from build123d import *

# Parameters (mm, degrees)
SKETCH1_W           = 87.952115464
SKETCH1_H           = 84
BOSS_EXTRUDE1_DEPTH = 44
CUT_EXTRUDE1_DEPTH  = 105.526999639
CUT_EXTRUDE2_DEPTH  = 94
BOSS_EXTRUDE2_DEPTH = 5
CUT_EXTRUDE4_DEPTH  = 108.023520294
BOSS_EXTRUDE3_DEPTH = 89
SKETCH12_W          = 66.643398472
SKETCH12_H          = 89
CUT_EXTRUDE5_DEPTH  = 21
SKETCH13_W          = 89
SKETCH13_H          = 4.850314153
CUT_EXTRUDE6_DEPTH  = 15
SKETCH14_R          = 9.5
CUT_EXTRUDE7_DEPTH  = 67.996371003
SKETCH15_R          = 4
SKETCH15_R_2        = 1.5
BOSS_EXTRUDE4_DEPTH = 5.5
CUT_EXTRUDE8_DEPTH  = 7
SKETCH17_R          = 32.5
CUT_EXTRUDE9_DEPTH  = 8


with BuildPart() as part:
    # Sketch1 → Boss-Extrude1 (new body)
    with BuildSketch(Plane(origin=(0, 0, 0), x_dir=(1, 0, 0), z_dir=(0, 1, 0))):
        Rectangle(SKETCH1_W, SKETCH1_H)
    extrude(amount=BOSS_EXTRUDE1_DEPTH)

    # Sketch3 → Cut-Extrude1 (cut, through all)
    with BuildSketch(Plane.XY.offset(42)):
        with BuildLine():
            Line((-21, 0), (21, 0))
            ThreePointArc((21, 0), (36.980443324, 19.654136956), (43.976057732, 44))
            Line((43.976057732, 44), (43.976057732, -11.97124173))
            Line((43.976057732, -11.97124173), (-43.976057732, -11.97124173))
            Line((-43.976057732, -11.97124173), (-43.976057732, 44))
            ThreePointArc((-43.976057732, 44), (-36.29063042, 20.014345617), (-21, 0))
        make_face()
    extrude(amount=-CUT_EXTRUDE1_DEPTH, mode=Mode.SUBTRACT)

    # Sketch4 → Cut-Extrude2 (cut)
    with BuildSketch(Plane.XY.offset(42)):
        with BuildLine():
            Line((-40.014597283, 44.55392338), (-43.976057732, 44))
            ThreePointArc((-43.976057732, 44), (-36.29063042, 20.014345617), (-21, 0))
            Line((-21, 0), (21, 0))
            ThreePointArc((21, 0), (36.980443324, 19.654136956), (43.976057732, 44))
            Line((43.976057732, 44), (39.988336247, 44.313173055))
            ThreePointArc((39.988336247, 44.313173055), (33.757294054, 22.132372023), (19.543536422, 4))
            Line((19.543536422, 4), (-19.406576645, 4))
            ThreePointArc((-19.406576645, 4), (-33.099796329, 22.554689448), (-40.014597283, 44.55392338))
        make_face()
    extrude(amount=-CUT_EXTRUDE2_DEPTH, mode=Mode.SUBTRACT)

    # Sketch6 → Boss-Extrude2 (add)
    with BuildSketch(Plane(origin=(0, 0, -42), x_dir=(-1, 0, 0), z_dir=(0, 0, -1))):
        with BuildLine():
            Line((-19.543536422, 4), (19.406576645, 4))
            ThreePointArc((19.406576645, 4), (32.972533813, 22.305488816), (39.934882496, 44))
            Line((39.934882496, 44), (-39.962906501, 44))
            ThreePointArc((-39.962906501, 44), (-33.686050128, 21.9923529), (-19.543536422, 4))
        make_face()
    extrude(amount=BOSS_EXTRUDE2_DEPTH)

    # Sketch8 → Cut-Extrude4 (cut, through all)
    with BuildSketch(Plane(origin=(0, 0, -47), x_dir=(-1, 0, 0), z_dir=(0, 0, -1))):
        with BuildLine():
            Line((-19.543536422, 4), (19.406576645, 4))
            ThreePointArc((19.406576645, 4), (20.408380664, 4.990013681), (21.390045584, 6))
            Line((21.390045584, 6), (-21.753352888, 6))
            ThreePointArc((-21.753352888, 6), (-20.661010919, 4.986115432), (-19.543536422, 4))
        make_face()
    extrude(amount=-CUT_EXTRUDE4_DEPTH, mode=Mode.SUBTRACT)

    # Sketch11 → Boss-Extrude3 (add)
    with BuildSketch(Plane(origin=(0, 0, -47), x_dir=(-1, 0, 0), z_dir=(0, 0, -1))):
        with BuildLine():
            Line((-21.753352888, 6), (21.390045584, 6))
            ThreePointArc((21.390045584, 6), (37.370443433, 22.115785334), (43.384826263, 44))
            Line((43.384826263, 44), (-44.615173737, 44))
            ThreePointArc((-44.615173737, 44), (-37.97109171, 22.12011544), (-21.753352888, 6))
        make_face()
    extrude(amount=-BOSS_EXTRUDE3_DEPTH)

    # Sketch12 → Cut-Extrude5 (cut)
    with BuildSketch(Plane.XZ.offset(-6)):
        with Locations((-4.068346348, -2.5)):
            Rectangle(SKETCH12_W, SKETCH12_H)
    extrude(amount=-CUT_EXTRUDE5_DEPTH, mode=Mode.SUBTRACT)

    # Sketch13 → Cut-Extrude6 (cut)
    with BuildSketch(Plane(origin=(-37.390045584, 0, 0), x_dir=(0, 0, -1), z_dir=(1, 0, 0))):
        with Locations((2.5, 24.574842924)):
            Rectangle(SKETCH13_W, SKETCH13_H)
    extrude(amount=-CUT_EXTRUDE6_DEPTH, mode=Mode.SUBTRACT)

    # Sketch14 → Cut-Extrude7 (cut, through all)
    with BuildSketch(Plane.XZ.offset(-27)):
        with Locations(Location((-23.812368574, 1, 0), (0, 0, 270))):
            Circle(SKETCH14_R)
    extrude(amount=-CUT_EXTRUDE7_DEPTH, mode=Mode.SUBTRACT)

    # Sketch15 → Boss-Extrude4 (add)
    # profile 1 of 3: a face of its own
    with BuildSketch(Plane.XZ.offset(-27)):
        with Locations(Location((-28.712368574, 37.1, 0), (0, 0, 90))):
            Circle(SKETCH15_R)
        with Locations(Location((-28.712368574, 37.1, 0), (0, 0, 270))):
            Circle(SKETCH15_R_2, mode=Mode.SUBTRACT)
    # profile 2 of 3: a face of its own
    with BuildSketch(Plane.XZ.offset(-27)):
        with Locations(Location((24.253352888, -0.4, 0), (0, 0, 90))):
            Circle(SKETCH15_R)
        with Locations(Location((24.253352888, -0.4, 0), (0, 0, 270))):
            Circle(SKETCH15_R_2, mode=Mode.SUBTRACT)
    # profile 3 of 3: a face of its own
    with BuildSketch(Plane.XZ.offset(-27)):
        with Locations(Location((-30.812368574, -34.8, 0), (0, 0, 90))):
            Circle(SKETCH15_R)
        with Locations(Location((-30.812368574, -34.8, 0), (0, 0, 270))):
            Circle(SKETCH15_R_2, mode=Mode.SUBTRACT)
    extrude(amount=BOSS_EXTRUDE4_DEPTH)

    # Sketch16 → Cut-Extrude8 (cut)
    with BuildSketch(Plane(origin=(0, 44, 0), x_dir=(1, 0, 0), z_dir=(0, 1, 0))):
        with BuildLine():
            Line((-9.884826263, -42), (11.615173737, -42))
            Line((11.615173737, -42), (11.615173737, -27))
            Line((11.615173737, -27), (24.115173737, -16))
            Line((24.115173737, -16), (24.115173737, 2.085392999))
            ThreePointArc((24.115173737, 2.085392999), (32.384099226, 20.131350652), (28.615173737, 39.620499352))
            Line((28.615173737, 39.620499352), (28.615173737, 47))
            Line((28.615173737, 47), (23.077098744, 47))
            ThreePointArc((23.077098744, 47), (-30.372036637, 35.259662676), (2.615173737, -8.403703492))
            Line((2.615173737, -8.403703492), (-9.884826263, -15))
            Line((-9.884826263, -15), (-9.884826263, -42))
        make_face()
    extrude(amount=-CUT_EXTRUDE8_DEPTH, mode=Mode.SUBTRACT)

    # Sketch17 → Cut-Extrude9 (cut)
    with BuildSketch(Plane(origin=(0, 37, 0), x_dir=(1, 0, 0), z_dir=(0, 1, 0))):
        with Locations((0.115173737, 24)):
            Circle(SKETCH17_R)
    extrude(amount=-CUT_EXTRUDE9_DEPTH, mode=Mode.SUBTRACT)


solid = part.part
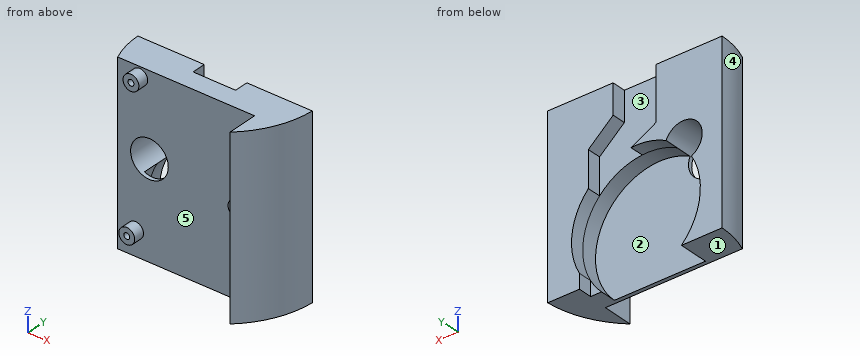
The model under review builds one solid part; all positions refer to its coordinate system, in mm. Face numbers are marked on the shaded views. A direction names the side the tool comes from. Give positions to 0.01 mm unless a question says otherwise; leave off trailing zeros. Order: outer loops, then holes, each group sorted by start corner. A loop starts at its lowest first (then second) coordinate and runs counter-clockwise, first axis right, second up. Notation, with made-up numbers: M -3,72 L 56,72 A24 cw 56,96 Z; hole C 77.25,89 d4. An arc over 180 degrees is marked long. Answer in a Markdown table with one row per item. Add a question column.
1. Add section D-D on z = 17.5. State the section outline as (x, y) points.
2. For pin 1 Ø2.5 at (x, z) = (-31, -34.5) entering from -Y; pin 2 Ø3.5 at (y, z) = (39.5, -43.5) entering from -X; pin 3 Ø10 at (y, z) = (28.5, -6) entering from +X, all flat-tipped, find the tip position at first contact; note any pin that passes through.
3. Add section A-A on y = 39. State the section outline as (x, z) points.
4. Add section C-C on z = 6. State the section outline as (x, y) points, plus the area to 3 significant figures.
5. Mouldability with a two-part tool opening along Z and no side actions: class the marked faces 1, 2 and 3 as released by +Z, released by -Z, zero draft, split by the parting line, or undercut.
6. To check wall thickness, follow line 1 along X through (y, z) = (25.45, 37.1); line 2 along X through (y, z) = (24, 38); line 3 along Y through (x, z) = (18.5, -35.5). State the ranges of each line that lie inside material, in increasing order.
7. Add section B-B on x = -20. State the section outline as (y, z) points.
8. Machinability: for the marked faces 4 and 5, which of the approach directions +Z, -Z, +X, -X, +Y, -Y give a long, thin tool a straight path to every point of the face, cutting with its end or side? Answer none if there is none.
The answers:
| question | item | result |
|---|---|---|
| 1 | outline | M -43.38,44 A44.73 ccw -39.81,27 L 29.25,27 L 29.25,11.53 A46.8 ccw 44.62,44 L 22.41,44 L 22.41,37 L -9.88,37 L -9.88,44 Z |
| 2 | pin 1 | y = 21.5 |
| 2 | pin 2 | x = -43.27 |
| 2 | pin 3 | x = 42.9 |
| 3 | outline | M -43.05,-47 L -22.85,-47 A32.5 cw -27.92,-7.56 A9.5 cw long -15.08,4.73 A32.5 cw 2.62,8.4 L -9.88,15 L -9.88,42 L -43.05,42 Z; M 11.62,27 L 24.12,16 L 24.12,-2.09 A32.5 cw 28.62,-39.62 L 28.62,-47 L 44.1,-47 L 44.1,42 L 11.62,42 Z |
| 4 | outline | M -43.38,44 A44.73 ccw -39.81,27 L -31.89,27 L -31.89,44 Z; M -15.73,27 L 29.25,27 L 29.25,11.53 A46.8 ccw 44.62,44 L 24.12,44 L 24.12,37 L 12.62,37 L 12.62,29 L -12.38,29 L -12.38,44 L -15.73,44 Z |
| 4 | area | 820 mm2 |
| 5 | face 1 | released by -Z |
| 5 | face 2 | undercut |
| 5 | face 3 | zero draft |
| 6 | line 1 | -32.71 to -30.21, -27.21 to -24.71, 29.25 to 39.79 |
| 6 | line 2 | -32.61 to -29.91, -27.51 to -24.81, 29.25 to 39.04 |
| 6 | line 3 | 27 to 29 |
| 7 | outline | M 27,-47 L 29,-47 L 29,-7.7 L 27,-7.7 Z; M 27,9.7 L 44,9.7 L 44,42 L 27,42 Z |
| 8 | face 4 | +Z, -Z, -X, -Y |
| 8 | face 5 | -Y |
